Geometry: final body of the model. Coordinates: model frame, mm. Give positions to 0.01 mm unless a question says otherwise; leave off trailing zeros. Write each loop counter-clockwise with the first axis right and the second up, starting at its lowest first coordinate (ties: lowest second). Pieces come first, ordered by that corner, then holes. Notation, with made-up numbers: (53, 62) -> (63, 62) arc R14 ccw to (63, 81) -> close; hole circle Ø4 at (-11, 28). An arc over 180 degrees is marked (long way). Answer in a Markdown table with one row per item. Add a question column.
Item 1: Material intervals for probe 1 along X at (y, z) = (8.25, 0.55); probe 2 along Y at (x, z) = (-2.5, 0.95), sorted ascending. Write a range as from..to.
Item 2: Section query B-B on x = 3.5. Output: boundary loops of the cut face in (y, z), plus the area to 3 significant figures.
Item 3: Section query A-A on z = 0.2. Output: boundary loops of the cut face in (x, y), plus the area to 3 significant figures.
Autodesk Inventor part; units mm, degrees
ref_plane "Start plane" through (0, 0, 0) normal (0, 0, 1) x (1, 0, 0)
ref_plane "End plane" through (0, 0, 1) normal (0, 0, 1) x (1, 0, 0)
ref_plane "YZ Plane" through (0, 0, 0) normal (1, 0, 0) x (0, 1, 0)
ref_plane "Start plane" through (0, 0, 0) normal (0, 0, 1) x (1, 0, 0)
ref_plane "End plane" through (0, 0, 1) normal (0, 0, 1) x (1, 0, 0)
sketch "Sketch2" plane through (0, 0, 0) normal (0, 0, 1) x (1, 0, 0)
  line L0 (-2.9751, 0.5249) -> (-2.9751, 12.2749)
  line L1 (-5.9751, 14.0249) -> (-4.7251, 14.0249)
  line L2 (-5.9751, -5.9751) -> (-5.9751, 14.0249)
  line L3 (-5.9751, -5.9751) -> (14.0249, -5.9751)
  line L4 (14.0249, -4.7251) -> (14.0249, -5.9751)
  line L5 (0.5249, -2.9751) -> (12.2749, -2.9751)
  arc A0 (-2.9751, 0.5249) -> (0.5249, -2.9751) centre (0.5249, 0.5249) ccw
  arc A1 (-2.9751, 12.2749) -> (-4.7251, 14.0249) centre (-4.7251, 12.2749) ccw
  arc A2 (14.0249, -4.7251) -> (12.2749, -2.9751) centre (12.2749, -4.7251) ccw
  line L6 (0, 60.8698) -> (0, -10.145) construction
  line L7 (-10.145, 0) -> (60.8698, 0) construction
  point P0 (-2.9751, -2.9751)
  point P1 (-2.9751, 14.0249)
  point P2 (14.0249, -2.9751)
  dimension "d4" = 20
  dimension "d6" = 20
  dimension "d8" = 3
  dimension "d10" = 3
  dimension "d17" = 3.5
  dimension "d18" = 1.75
  dimension "d19" = 5.9751
  dimension "d20" = 5.9751
extrude "Body" add sketch "Sketch2" along normal up to surface (1 mm away) from surface at 0
sketch "Sketch3" plane through (0, 0, 0) normal (0, 0, 1) x (1, 0, 0)
  line L0 (0, 0) -> (10, 0)
ref_plane "Work Plane10" through (0, 0, 0) normal (0, -1, 0) x (1, 0, 0)
sketch "Sketch4" plane through (0, 0, 0) normal (0, -1, 0) x (1, 0, 0)
  line L0 (-2, 0) -> (12, 0)
  line L1 (-2, 1) -> (12, 1)
  dimension "d24" = 1
equation "\"d4\" = b"
equation "\"d6\" = b"
equation "\"d17\" = R"
equation "\"d18\" = R1"
equation "\"d19\" = ex"
equation "\"d20\" = d19"
equation "\"d11\" = G_L"
equation "\"b\" = 20"
equation "\"ParT\" = 3"
equation "\"R\" = 3.5"
equation "\"R1\" = 1.75"
equation "\"G_L\" = d24"
equation "\"G_OFFSET_START\" = 0"
equation "\"G_OFFSET_END\" = 0"
equation "\"d22\" = G_OFFSET_END + B_L"
equation "\"B_L\" = 1"
properties part number "STN EN 10056-1 - L20x20x3-1" material "鋼、軟鋼"
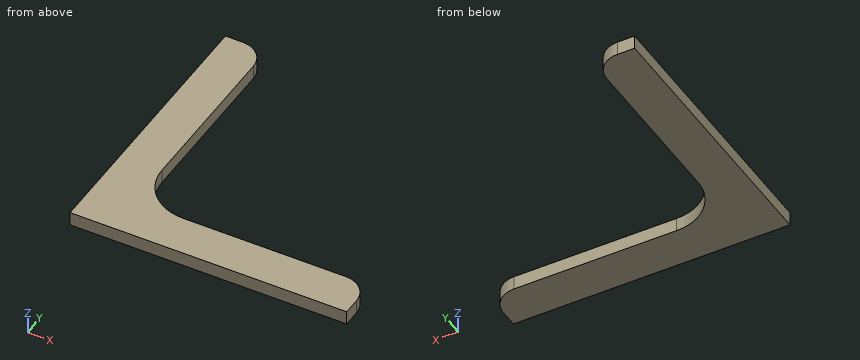
Findings below:
| question | item | result |
|---|---|---|
| 1 | probe 1 | x = -5.98..-2.98 |
| 1 | probe 2 | y = -5.98..-1.24 |
| 2 | outline | (-5.98, 0) -> (-2.98, 0) -> (-2.98, 1) -> (-5.98, 1) -> close |
| 2 | area | 3.00 mm^2 |
| 3 | outline | (-5.98, -5.98) -> (14.02, -5.98) -> (14.02, -4.73) arc R1.75 ccw to (12.27, -2.98) -> (0.52, -2.98) arc R3.5 cw to (-2.98, 0.52) -> (-2.98, 12.27) arc R1.75 ccw to (-4.73, 14.02) -> (-5.98, 14.02) -> close |
| 3 | area | 112 mm^2 |
